The figure shows three views and two pictorial views of one solid part (mm, origin at its lowest corner). Answer the questions. A direction names the side the tool comes from. Round coordinates to 2 decimals unless told otherwise and drop trailing zeros. Order: outer loops, then holes, each group sorted by start corner. A loop starts at its lowest first (then second) coordinate and runs counter-clockwise, first axis right, second up. Notation, with made-up numbers: (86, 32.5) - (94, 32.5) arc R34 cw to (94, 66.5) - close; hole circle Ø5 at (-21, 36.5). An arc over 180 degrees is marked (long way). Answer as a JSON object with one key per item and string values. Group by question number.
Q1. A tool of negligible diameter and unlimited length cuts with its end or side. For the marked faces 4 and 5, from which of +Z, -Z, +X, -X, +Y, -Y can it reach the whole face along a straight path? Write none if from no direction.
Q2. Given pin 1 Ø5 at (y, z) = (7.5, 10) entering from +X; pin 2 Ø1.5 at (x, z) = (21.5, 7.5) entering from +Y, each flat-ended and moving along its own axis, determine where each tip first touches the part or whether it passes through.
Q3. The mould has two halves that part along Y. Classify the marked faces 1, 2 and 3: pulls with the +Y half, pulls with the -Y half, needs draft (parallel to the pull), parting line crosses it, or undercut.
Q4. A cutting plane is placed at B-B on y = 35. Determine the outline of the cut face in (x, z).
Q5. A cutting plane is placed at D-D on z = 3. Determine the outline of the cut face in (x, y) (3 decimals), and give its area (3 significant figures).
Q6. Consider line 1 (Z direction, x = 27.5, y = 60.5); line 2 (Y direction, x = 35, z = 2.25); line 3 (X direction, y = 24.5, z = 3). Determine where each line is inside the solid, lowest interval first.
Q7. A cutting plane is placed at A-A on x = 49. Determine the outline of the cut face in (y, z).
Q8. A cutting plane is placed at C-C on y = 12.5. Determine the outline of the cut face in (x, z).
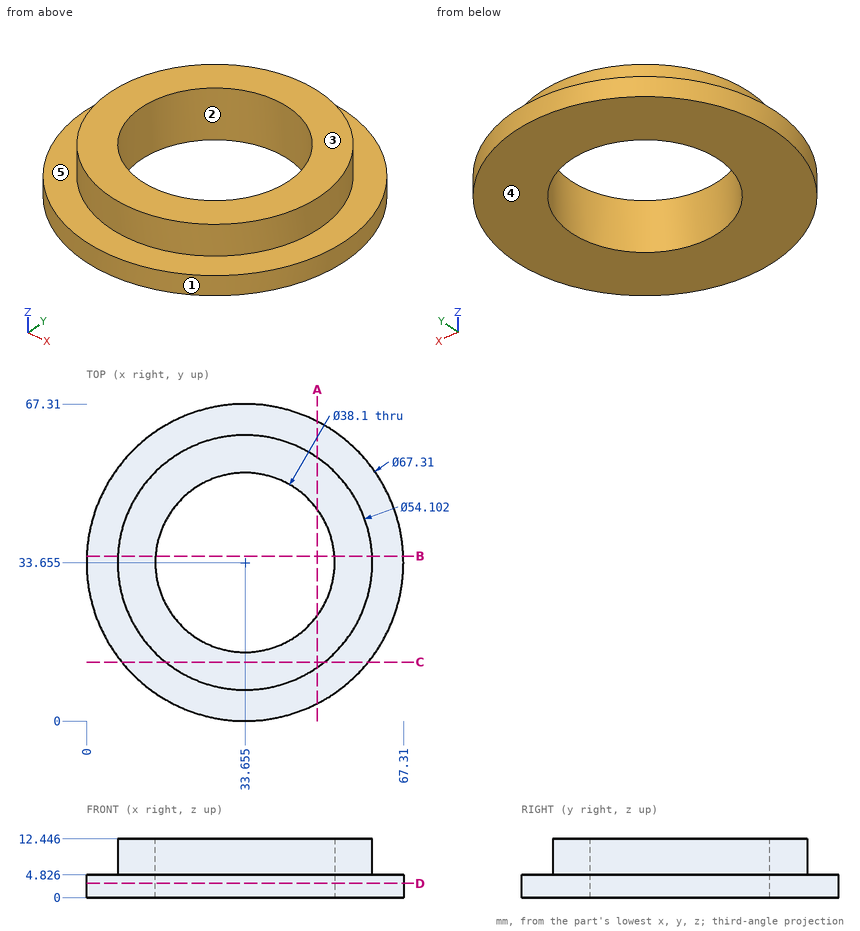
Result set:
{
 "1": {"face 4": "-Z, +X, -X, +Y, -Y", "face 5": "+Z"},
 "2": {"pin 1": "stops at x = 46.78", "pin 2": "stops at y = 58.18"},
 "3": {"face 1": "parting line crosses it", "face 2": "undercut", "face 3": "needs draft"},
 "4": {"outline": "(0.03, 0) - (14.65, 0) - (14.65, 12.45) - (6.64, 12.45) - (6.64, 4.83) - (0.03, 4.83) - close; (52.66, 0) - (67.28, 0) - (67.28, 4.83) - (60.67, 4.83) - (60.67, 12.45) - (52.66, 12.45) - close"},
 "5": {"outline": "circle Ø67.31 at (33.655, 33.655); hole circle Ø38.1 at (33.655, 33.655)", "area": "2,420 mm²"},
 "6": {"line 1": "z = 0 to 4.83", "line 2": "y = 0.03 to 14.65, 52.66 to 67.28", "line 3": "x = 1.27 to 16.95, 50.36 to 66.04"},
 "7": {"outline": "(3.7, 0) - (22.37, 0) - (22.37, 12.45) - (11.38, 12.45) - (11.38, 4.83) - (3.7, 4.83) - close; (44.94, 0) - (63.61, 0) - (63.61, 4.83) - (55.93, 4.83) - (55.93, 12.45) - (44.94, 12.45) - close"},
 "8": {"outline": "(7.48, 0) - (59.83, 0) - (59.83, 4.83) - (50.51, 4.83) - (50.51, 12.45) - (16.8, 12.45) - (16.8, 4.83) - (7.48, 4.83) - close"}
}
